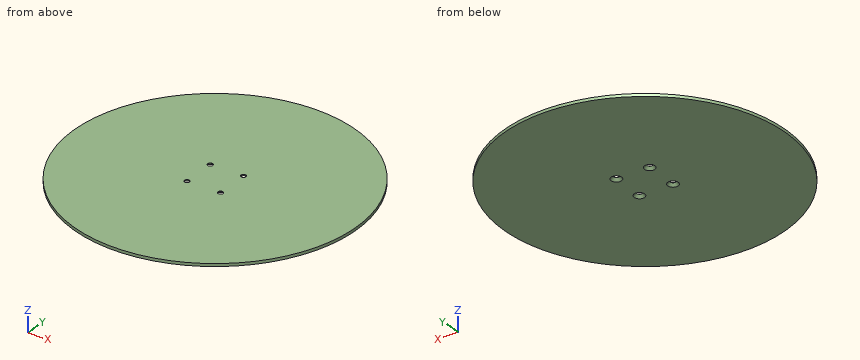
```python
from build123d import *

# Parameters (mm, degrees)
SKETCH1_R                    = 150
BOSS_EXTRUDE1_DEPTH          = 3
CSK_FOR_M5_SFHCS1_AT_2_COUNT = 2
CSK_FOR_M5_SFHCS1_AT_2_PITCH = 35.289297711
CSK_FOR_M5_SFHCS1_AT_3_COUNT = 2
CSK_FOR_M5_SFHCS1_AT_3_PITCH = 50.17586669
CSK_FOR_M5_SFHCS1_AT_4_COUNT = 2
CSK_FOR_M5_SFHCS1_AT_4_PITCH = 35.678748885


with BuildPart() as part:
    # Sketch1 → Boss-Extrude1 (new body)
    with BuildSketch(Plane.XY):
        Circle(SKETCH1_R)
    extrude(amount=BOSS_EXTRUDE1_DEPTH)

    # Sketch4 → CSK for M5 SFHCS1 (revolve, cut)
    with BuildSketch(Plane(origin=(17.080766051, 18.586987198, 0), x_dir=(0, 1, 0), z_dir=(1, 0, 0))):
        Polygon((0, 0), (0, 3), (2.75, 3), (2.75, 2.85), (5.6, 0), align=None)
    csk_for_m5_sfhcs1 = revolve(axis=Axis((17.080766051, 18.586987198, -6.35), (0, 0, 1)), mode=Mode.SUBTRACT)

    # CSK for M5 SFHCS1 at 2: CSK for M5 SFHCS1 ×2
    with Locations(*[Vector(-0.99906632, -0.043202868, 0) * (i * CSK_FOR_M5_SFHCS1_AT_2_PITCH) for i in range(1, CSK_FOR_M5_SFHCS1_AT_2_COUNT)]):
        add(csk_for_m5_sfhcs1, mode=Mode.SUBTRACT)

    # CSK for M5 SFHCS1 at 3: CSK for M5 SFHCS1 ×2
    with Locations(*[Vector(-0.676068537, -0.736838743, 0) * (i * CSK_FOR_M5_SFHCS1_AT_3_PITCH) for i in range(1, CSK_FOR_M5_SFHCS1_AT_3_COUNT)]):
        add(csk_for_m5_sfhcs1, mode=Mode.SUBTRACT)

    # CSK for M5 SFHCS1 at 4: CSK for M5 SFHCS1 ×2
    with Locations(*[Vector(0.048072698, -0.998843839, 0) * (i * CSK_FOR_M5_SFHCS1_AT_4_PITCH) for i in range(1, CSK_FOR_M5_SFHCS1_AT_4_COUNT)]):
        add(csk_for_m5_sfhcs1, mode=Mode.SUBTRACT)


solid = part.part
```
Could you check a few things on this model? Use its own coordinates, in mm. Coordinates: 2 decimals unless noted, no trailing zeros. Write each loop counter-clockwise with the first axis right and the second up, starting at its lowest first coordinate (ties: lowest second). Pieces come first, ordered by that corner, then holes. Notation, with made-up numbers: (14, 86) -> (18, 86) arc R22 cw to (18, 100) -> close; hole circle Ø5 at (9, 84.5). An arc over 180 degrees is marked (long way). Write item = value, one per line. Start each with the question number.
(1) I want a section at B-B (x = 58.5). Please give me the cut outline in (y, z).
(2) I need wall thicknesses on line 1 (Y direction, x = -15, z = 1.65); line 2 (X direction, y = -18, z = 0.75); line 3 (Y direction, x = 16, z = 0.5). Which ranges of each line are inside material? Lowest first, please. Write a range as [from, to].
(3) I want a section at A-A (z = 1.7). Please give me the cut outline in (x, y).
(4) I want a section at C-C (y = -65). Please give me the cut outline in (x, z), plus the area to 3 significant figures.
(5) Will this pin go through, and if not, where does the flat tip stop? pin 1 (5 mm diameter, centred on x = 18.8, y = -17.05, fed in from +Z).
Result set:
q1.outline = (-138.12, 0) -> (138.12, 0) -> (138.12, 3) -> (-138.12, 3) -> close
q2.line_1 = [-149.25, -21.88], [-14.89, 14.71], [19.41, 149.25]
q2.line_2 = [-148.92, -21.68], [-12.01, 14.04], [23.55, 148.92]
q2.line_3 = [-149.14, -21.32], [-12.79, 13.6], [23.57, 149.14]
q3.outline = circle Ø300 at (0, 0); hole circle Ø7.8 at (-18.18, 17.06); hole circle Ø7.8 at (-16.84, -18.38); hole circle Ø7.8 at (17.08, 18.59); hole circle Ø7.8 at (18.8, -17.05)
q4.outline = (-135.19, 0) -> (135.19, 0) -> (135.19, 3) -> (-135.19, 3) -> close
q4.area = 811 mm2
q5.pin_1 = through
